The figure shows three views and two pictorial views of one solid part (mm, origin at its lowest corner). Answer the questions. A direction names the side the tool comes from. Give positions to 0.01 mm unless a question says otherwise; leave off trailing zeros. Loops run counter-clockwise (first coordinate to the right, second up) from the corner with the lowest first, then second, coordinate; pieces in that order, holes last. Notation, with made-up numbers: (12, 88) - (44, 88) arc R24 ccw to (44, 121) - close; hole circle Ø7 at (9.25, 84.5). An arc over 180 degrees is marked (long way). Use CSV: the item, a comma, the result in double quotes.
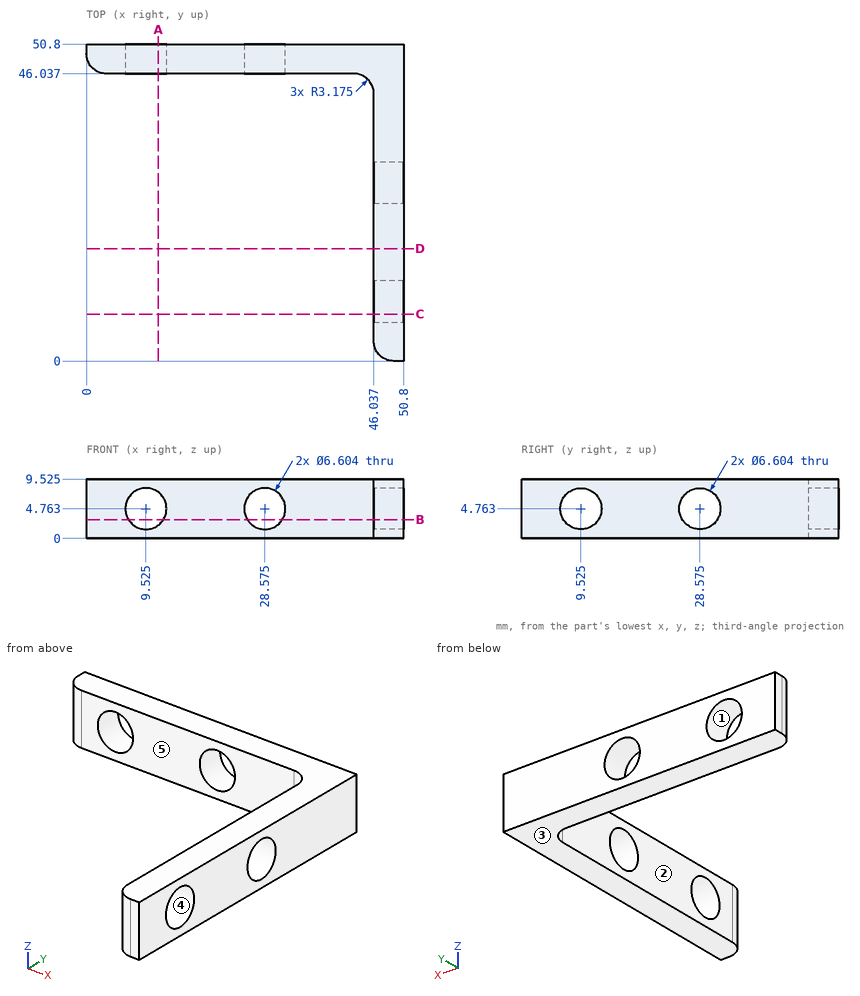
Item 1: A cutting plane is placed at B-B on z = 3. State how many separate pieces and enclosed holes the cut face has.
Determined:
separate pieces,"5"
enclosed holes,"0"
Item 2: Given P1, Ø3, axis at y = 5.5, z = 7, coming from the -X side, flat-ended and moving along its own axis, determine where the tip first touches the part or whether it passes through.
Determined:
P1,"stops at x = 46.04"
Item 3: For the marked faces 4 and 5, determine the directions among +Z, -Z, +X, -X, +Y, -Y from which every point of the face is accessible in a straight line to the end or side of a thin tool.
Determined:
face 4,"+X, -X"
face 5,"+Z, -Z, -X, -Y"
Item 4: A cutting plane is placed at D-D on y = 18. Determine the outline of the cut face in (x, z) (1 decimal).
Determined:
outline,"(46, 0) - (50.8, 0) - (50.8, 9.5) - (46, 9.5) - close"
Item 5: Find the intervals of material crossed by line 1 (Y direction, x = 33.5, z = 1); line 2 (Y direction, x = 48, z = 1), in increasing order.
Determined:
line 1,"y = 46.04 to 50.8"
line 2,"y = 0.24 to 50.8"
Item 6: A cutting plane is placed at A-A on x = 11.5. Determine the outline of the cut face in (y, z) (1 decimal).
Determined:
outline,"(46, 0) - (50.8, 0) - (50.8, 2.1) - (46, 2.1) - close; (46, 7.4) - (50.8, 7.4) - (50.8, 9.5) - (46, 9.5) - close"
Item 7: The mould has two halves that part along Z. Classify the marked faces 1, 2 and 3: pulls with the +Z half, pulls with the -Z half, needs draft (parallel to the pull), parting line crosses it, or undercut.
Determined:
face 1,"undercut"
face 2,"needs draft"
face 3,"pulls with the -Z half"
Item 8: A cutting plane is placed at C-C on y = 7.5. Determine the outline of the cut face in (x, z) (1 decimal), and give its area (3 significant figures).
Determined:
outline,"(46, 0) - (50.8, 0) - (50.8, 2.2) - (46, 2.2) - close; (46, 7.4) - (50.8, 7.4) - (50.8, 9.5) - (46, 9.5) - close"
area,"20.5 mm²"
